from build123d import *

# Parameters (mm, degrees)
SKETCH_R     = 4
PAD_DEPTH    = 41
FILLET_R     = 4
PAD001_DEPTH = 6
SKETCH002_R  = 3.75
PAD002_DEPTH = 2.5
PAD003_DEPTH = 7.5
SKETCH004_R  = 1
PAD004_DEPTH = 10


with BuildPart() as part:
    # Sketch → Pad (new body)
    with BuildSketch(Plane.YZ):
        Circle(SKETCH_R)
    extrude(amount=PAD_DEPTH)

    # Fillet
    fillet_edges = [part.edges().sort_by_distance(p)[0] for p in [
        (41, -4, 0),
    ]]
    fillet(fillet_edges, radius=FILLET_R)

    # Sketch001 (on Face3 of Fillet) → Pad001 (join)
    with BuildSketch(Plane(origin=(0, 0, 0), x_dir=(0, 1, 0), z_dir=(-1, 0, 0))):
        Polygon((4.618802, 0), (2.309401, 4), (-2.309401, 4), (-4.618802, 0), (-2.309401, -4), (2.309401, -4), align=None)
    extrude(amount=PAD001_DEPTH)

    # Sketch002 (on Face15 of Pad001) → Pad002 (join)
    with BuildSketch(Plane(origin=(-6, 0, 0), x_dir=(0, 1, 0), z_dir=(-1, 0, 0))):
        Circle(SKETCH002_R)
    extrude(amount=PAD002_DEPTH)

    # Sketch003 (on Face17 of Pad002) → Pad003 (join)
    with BuildSketch(Plane(origin=(-8.5, 0, 0), x_dir=(0, 1, 0), z_dir=(-1, 0, 0))):
        Polygon((4.907477, 0), (2.453739, 4.25), (-2.453739, 4.25), (-4.907477, 0), (-2.453739, -4.25), (2.453739, -4.25), align=None)
    extrude(amount=PAD003_DEPTH)

    # Sketch004 (on Face24 of Pad003) → Pad004 (join)
    with BuildSketch(Plane(origin=(-16, 0, 0), x_dir=(0, 1, 0), z_dir=(-1, 0, 0))):
        Circle(SKETCH004_R)
    extrude(amount=PAD004_DEPTH)


solid = part.part
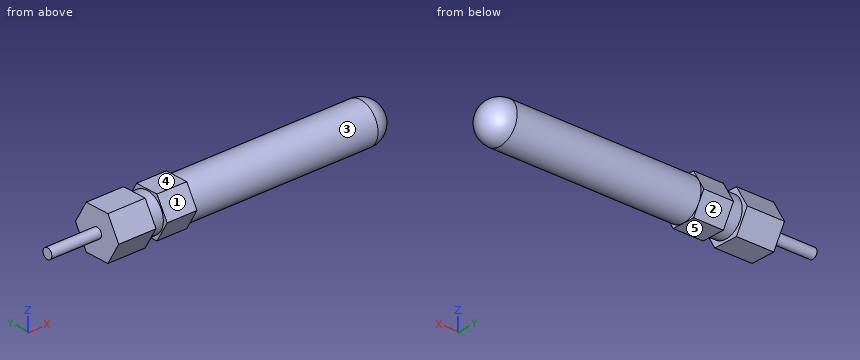
For this review, take the finished solid that the model builds, in its own axes (mm). Face numbers are marked on the shaded views. A direction names the side the tool comes from. Give positions to 0.01 mm unless a question says otherwise; leave off trailing zeros. Order: outer loops, then holes, each group sorted by start corner. A loop starts at its lowest first (then second) coordinate and runs counter-clockwise, first axis right, second up. Notation, with made-up numbers: (-26.5, -26.75) - (1.5, -26.75) arc R14 cw to (1.5, -17.75) - close; hole circle Ø2 at (75, 9). An arc over 180 degrees is marked (long way). Answer as a JSON object with one key per item and string values. Group by question number.
Item 1: Wall thickness on line 1 along X through (y, z) = (2.75, -3); line 2 along Z through (x, y) = (18.5, 2): over which ranges is each line inside the solid? List them lowest first.
Item 2: Take a section at B-B on y = 1.75. Give the boundary of the cut face in (x, z), and give its area (3 significant figures).
Item 3: Take a section at C-C on x = 23.5. Give the boundary of the cut face in (y, z).
Item 4: Clearance check with flat-ended pins moving along their axes: pin 1 Ø1.5 at (y, z) = (2.5, -1.5) entering from -X; pin 2 Ø0.6 at (y, z) = (1.5, -3) entering from +X; pin 3 Ø2.5 at (x, y) = (-3.5, 1) entering from -Z. State where each tip first meets the part, or that it passes through.
Item 5: Machinability: for the marked faces 1, 2, 3, 4 and 5, which of the approach directions +Z, -Z, +X, -X, +Y, -Y give a long, thin tool a straight path to every point of the face, cutting with its end or side? Answer none if there is none.
Item 6: Take a section at A-A on x = -3.5. Give the boundary of the cut face in (y, z).
Reported:
{
 "1": {"line 1": "-16 to -8.5, -6 to 0", "line 2": "-3.46 to 3.46"},
 "2": {"outline": "(-16, -4.25) - (-8.5, -4.25) - (-8.5, -3.32) - (-6, -3.32) - (-6, -4) - (0, -4) - (0, -3.6) - (37, -3.6) arc R3.6 ccw to (37, 3.6) - (0, 3.6) - (0, 4) - (-6, 4) - (-6, 3.32) - (-8.5, 3.32) - (-8.5, 4.25) - (-16, 4.25) - close", "area": "415 mm^2"},
 "3": {"outline": "circle Ø8 at (0, 0)"},
 "4": {"pin 1": "x = -16", "pin 2": "x = 39.58", "pin 3": "z = -4"},
 "5": {"face 1": "+Z, +X, -Y", "face 2": "-Z, +X, +Y", "face 3": "+X", "face 4": "+Z, +X, +Y, -Y", "face 5": "-Z, +X, +Y, -Y"},
 "6": {"outline": "(-4.62, 0) - (-2.31, -4) - (2.31, -4) - (4.62, 0) - (2.31, 4) - (-2.31, 4) - close"}
}
